```python
from build123d import *

# Parameters (mm, degrees)
BOSS_EXTRUDE1_DEPTH      = 3
BOSS_EXTRUDE1_DEPTH_BACK = 3


with BuildPart() as part:
    # Sketch1 → Boss-Extrude1 (new body, two sides)
    with BuildSketch(Plane.XY.offset(25.67)) as boss_extrude1_sk:
        with BuildLine():
            Line((60.116638829, -51.1464666), (8.633428278, -25.015226292))
            ThreePointArc((8.633428278, -25.015226292), (-18.470533149, -37.260691846), (-0.670439202, -61.087836182))
            Line((-0.670439202, -61.087836182), (57.029169306, -63.117088912))
            ThreePointArc((57.029169306, -63.117088912), (63.381062097, -58.371900532), (60.116638829, -51.1464666))
        make_face()
        with BuildLine():
            Line((60.003487737, -51.369394459), (8.520277187, -25.238154151))
            ThreePointArc((8.520277187, -25.238154151), (-18.228455389, -37.323128676), (-0.661652319, -60.837990648))
            Line((-0.661652319, -60.837990648), (57.037956189, -62.867243378))
            ThreePointArc((57.037956189, -62.867243378), (63.138984336, -58.309463702), (60.003487737, -51.369394459))
        make_face(mode=Mode.SUBTRACT)
    extrude(amount=BOSS_EXTRUDE1_DEPTH)
    extrude(boss_extrude1_sk.sketch, amount=-BOSS_EXTRUDE1_DEPTH_BACK)


solid = part.part
```
Could you check a few things on this model? Use its own coordinates, in mm. Coordinates: 2 decimals unless noted, no trailing zeros. Order: outer loops, then holes, each group sorted by start corner. A loop starts at its lowest first (then second) coordinate and runs counter-clockwise, first axis right, second up. Notation, with made-up numbers: M 4,57 L 44,57 A27 ccw 44,85 Z; hole C -16.75,28 d8. An arc over 180 degrees is marked long. Use one line per item in the form item = value. Start each with the question number.
1. Please list where these lines run through material, in increasing order: line 1 (X direction, y = -54, z = 26.75); line 2 (X direction, y = -28.5, z = 23.8); line 3 (Y direction, x = 0, z = 25.35).
2. Suppose I cut it at A-A on z = 26.45. Write out the boundary of the cut face in (x, y) (3 decimals), then the cut area to 3 significant figures.
3. For pin 1 (1 mm diameter, centred on x = -3.5, z = 23.5, fed in from -Y); pin 2 (3 mm diameter, centred on x = 15.5, z = 24, fed in from -Y); pin 3 (1.5 mm diameter, centred on x = 8.5, z = 26, fed in from +Y), each with a flat end and sliding along its axis, tell me the tip position at first contact or that it passes through.
4. We'd pull the mould along X, two halves only. Please class faces 1 (the flat face through (34.622, -38.487, 25.712)), 2 (the flat face through (34.735, -38.264, 25.712)): +X half, -X half, draft (parallel to the pull), parting line (faces both ways), or undercut.
5. Suppose I cut it at B-B on x = 20. Write out the boundary of the cut face in (y, z), then the cut area to 3 significant figures.
6. Suppose I cut it at C-C on x = -3. Write out the boundary of the cut face in (y, z), then the cut area to 3 significant figures.
Geometry says:
q1.line_1 = -14.85 to -14.52, 62.65 to 62.93
q1.line_2 = -13.45 to -13.09, 14.95 to 15.5
q1.line_3 = -61.11 to -60.86, -23.2 to -22.95
q2.outline = M -0.67,-61.088 L 57.029,-63.117 A6.33 ccw 60.117,-51.146 L 8.633,-25.015 A19.075 ccw long Z; hole M -0.662,-60.838 L 57.038,-62.867 A6.08 ccw 60.003,-51.369 L 8.52,-25.238 A18.825 ccw long Z
q2.area = 50.0 mm^2
q3.pin_1 = -60.86
q3.pin_2 = -61.71
q3.pin_3 = -24.59
q4.face_1 = undercut
q4.face_2 = +X half
q5.outline = M -61.81,22.67 L -61.56,22.67 L -61.56,28.67 L -61.81,28.67 Z; M -31.06,22.67 L -30.78,22.67 L -30.78,28.67 L -31.06,28.67 Z
q5.area = 3.18 mm^2
q6.outline = M -60.86,22.67 L -60.61,22.67 L -60.61,28.67 L -60.86,28.67 Z; M -23.44,22.67 L -23.19,22.67 L -23.19,28.67 L -23.44,28.67 Z
q6.area = 3.04 mm^2
